Geometry check sheet. Reference: the model listing, model coordinates, mm. A direction names the side the tool comes from. Coordinates: 2 decimals unless noted, no trailing zeros. Write each loop counter-clockwise with the first axis right and the second up, starting at its lowest first coordinate (ties: lowest second). Pieces come first, ordered by that corner, then holes. Notation, with made-up numbers: (34.25, -19.75) -> (57.25, -19.75) arc R27 ccw to (57.25, 8.25) -> close; hole circle Ø7 at (40.25, -22). An arc over 180 degrees is marked (long way). One line per question, with ' | ' between items.
```python
from build123d import *

# Parameters (mm, degrees)
SKETCH_2_R      = 1.985
SKETCH_2_R_2    = 44.910539349
EXTRUDE_1_DEPTH = 1


with BuildPart() as part:
    # 草图1 → 旋转1 (revolve)
    with BuildSketch(Plane.XY, mode=Mode.PRIVATE) as revolve_1_sk:
        with BuildLine():
            ThreePointArc((-45.813874016, -0.428936451), (-43.539426354, -2.86488143), (-40.275857757, -3.540203663))
            ThreePointArc((-40.275857757, -3.540203663), (-35.905809817, -1.000028754), (-31.553091654, -3.569785971))
            Line((-31.553091654, -3.569785971), (-27, -3.569785971))
            Line((-27, -3.569785971), (-27, -2.569785971))
            Line((-27, -2.569785971), (-31, -2.569785971))
            ThreePointArc((-31, -2.569785971), (-35.922766673, 0), (-40.845533346, -2.569785971))
            ThreePointArc((-40.845533346, -2.569785971), (-43.250116145, -1.873465974), (-44.910539349, 0))
            Line((-44.910539349, 0), (-45.813874016, -0.428936451))
        make_face()
    revolve(revolve_1_sk.sketch.rotate(Axis((0, 6.917160425, 0), (0, -1, 0)), 270), axis=Axis((0, 6.917160425, 0), (0, -1, 0)))

    # 草图2 → 凸台-拉伸1 (add)
    with BuildSketch(Plane(origin=(0, 0, 0), x_dir=(1, 0, 0), z_dir=(0, 1, 0))):
        with BuildLine():
            Line((46.8, 50.8), (-46.8, 50.8))
            ThreePointArc((-46.8, 50.8), (-49.628427125, 49.628427125), (-50.8, 46.8))
            Line((-50.8, 46.8), (-50.8, -46.8))
            ThreePointArc((-50.8, -46.8), (-49.628427125, -49.628427125), (-46.8, -50.8))
            Line((-46.8, -50.8), (46.8, -50.8))
            ThreePointArc((46.8, -50.8), (49.628427125, -49.628427125), (50.8, -46.8))
            Line((50.8, -46.8), (50.8, 46.8))
            ThreePointArc((50.8, 46.8), (49.628427125, 49.628427125), (46.8, 50.8))
        make_face()
        with Locations(Location((-44.845, -44.845, 0), (0, 0, 270))):
            Circle(SKETCH_2_R, mode=Mode.SUBTRACT)
        with Locations(Location((44.845, -44.845, 0), (0, 0, 270))):
            Circle(SKETCH_2_R, mode=Mode.SUBTRACT)
        Circle(SKETCH_2_R_2, mode=Mode.SUBTRACT)
        with Locations(Location((-44.845, 44.845, 0), (0, 0, 270))):
            Circle(SKETCH_2_R, mode=Mode.SUBTRACT)
        with Locations(Location((44.845, 44.845, 0), (0, 0, 270))):
            Circle(SKETCH_2_R, mode=Mode.SUBTRACT)
    extrude(amount=-EXTRUDE_1_DEPTH)


solid = part.part
```
(1) Tool access check on faces 1 (the face through (-46, -1, -1)), 2 (the face through (-46, 0, -1)), 3 (the face through (-28, -2.57, -2)). Record the directions out of +Z, -Z, +X, -X, +Y, -Y that give a thin tool (end or side, any length) a straight path to the whole face; none if there is none.
Answers below:
face 1: -Y | face 2: +Z, -Z, +X, -X, +Y | face 3: +Y
(2) Cross-section at A-A (z = 0). Record the cut outline in (x, y), plus the area to 3 significant figures.
Answers below:
outline: (-50.8, -1) -> (-45.5, -1) arc R5.5 ccw to (-40.28, -3.54) arc R5 cw to (-31.55, -3.57) -> (-27, -3.57) -> (-27, -2.57) -> (-31, -2.57) arc R6 ccw to (-40.85, -2.57) arc R4.5 cw to (-44.91, 0) -> (-50.8, 0) -> close; (27, -3.57) -> (31.55, -3.57) arc R5 cw to (40.28, -3.54) arc R5.5 ccw to (45.5, -1) -> (50.8, -1) -> (50.8, 0) -> (44.91, 0) arc R4.5 cw to (40.85, -2.57) arc R6 ccw to (31, -2.57) -> (27, -2.57) -> close | area: 53.1 mm²
(3) Depth check by flat-ended pin: P1, Ø5, axis at x = 44.845, z = -44.845, coming from the -Y side; P2, Ø10, axis at x = -24, z = -4, coming from the -Y side; P3, Ø4, axis at x = -20.5, z = -13, coming from the -Y side. Enter the tip coordinate at first touch or a pass-through.
Answers below:
P1: stops at y = -1 | P2: stops at y = -3.57 | P3: passes through
(4) Cross-section at C-C (y = -2). Record the cut outline in (x, z), plus the area to 3 significant figures.
Answers below:
outline: circle Ø89.39 at (0, 0); circle Ø80.79 at (0, 0); circle Ø65.85 at (0, 0); hole circle Ø86.07 at (0, 0); hole circle Ø77.85 at (0, 0); hole circle Ø62.9 at (0, 0) | area: 1,120 mm²
(5) Material ranges on line 1 (X direction, y = -1.85, z = -13); line 2 (Z direction, x = 1, y = -1.85); line 3 (Z direction, x = 46, y = -0.9), recorded low to high.
Answers below:
line 1: x = -42.91 to -41.29, -38.1 to -36.46, -30.48 to -28.79, 28.79 to 30.48, 36.46 to 38.1, 41.29 to 42.91 | line 2: z = -44.83 to -43.28, -40.24 to -38.7, -33.12 to -31.57, 31.57 to 33.12, 38.7 to 40.24, 43.28 to 44.83 | line 3: z = -50.8 to -46.46, -43.23 to 43.23, 46.46 to 50.8
(6) Cross-section at B-B (x = 0). Record the cut outline in (y, z).
Answers below:
outline: (-3.57, -31.55) arc R5 cw to (-3.54, -40.28) arc R5.5 ccw to (-1, -45.5) -> (-1, -50.8) -> (0, -50.8) -> (0, -44.91) arc R4.5 cw to (-2.57, -40.85) arc R6 ccw to (-2.57, -31) -> (-2.57, -27) -> (-3.57, -27) -> close; (-3.57, 27) -> (-2.57, 27) -> (-2.57, 31) arc R6 ccw to (-2.57, 40.85) arc R4.5 cw to (0, 44.91) -> (0, 50.8) -> (-1, 50.8) -> (-1, 45.5) arc R5.5 ccw to (-3.54, 40.28) arc R5 cw to (-3.57, 31.55) -> close
(7) Draft check along Z on faces 4 (the face through (-49.659, -0.493, 49.597)), 5 (the face through (46.187, -0.493, 43.382)), 6 (the face through (-14.2, -3.57, 23.2)). Enter one of: pulls with the +Z half, pulls with the -Z half, needs draft (parallel to the pull), parting line crosses it, or undercut.
Answers below:
face 4: pulls with the +Z half | face 5: undercut | face 6: needs draft
